from build123d import *

# Parameters (mm, degrees)
SKETCH1_W              = 215
SKETCH1_H              = 49
BOSS_EXTRUDE1_DEPTH    = 6
CUT_EXTRUDE1_REACH     = 141.058
SKETCH2_W              = 72
SKETCH2_H              = 6
SKETCH2_W_2            = 117
M8X1_25_TAPPED_HOLE1_D = 6.8
CUT_EXTRUDE2_REACH     = 141.058
SKETCH5_W              = 6
SKETCH5_H              = 20
SKETCH6_W              = 100
SKETCH6_H              = 6
BOSS_EXTRUDE2_DEPTH    = 6


with BuildPart() as part:
    # Sketch1 → Boss-Extrude1 (new body)
    with BuildSketch(Plane.XY):
        with Locations((-22.5, 24.5)):
            Rectangle(SKETCH1_W, SKETCH1_H)
    extrude(amount=BOSS_EXTRUDE1_DEPTH)

    # Sketch2 → Cut-Extrude1 (cut, up to next)
    with BuildSketch(Plane(origin=(0, 0, 0), x_dir=(-1, 0, 0), z_dir=(0, 0, -1)), mode=Mode.PRIVATE) as cut_extrude1_sk1:
        with Locations((-49, 46)):
            Rectangle(SKETCH2_W, SKETCH2_H)
    cut_extrude1_tool1 = extrude(cut_extrude1_sk1.sketch, amount=-CUT_EXTRUDE1_REACH, mode=Mode.PRIVATE) & part.part
    # Sketch2 → Cut-Extrude1 (cut, up to next)
    with BuildSketch(Plane(origin=(0, 0, 0), x_dir=(-1, 0, 0), z_dir=(0, 0, -1)), mode=Mode.PRIVATE) as cut_extrude1_sk2:
        with Locations((71.5, 46)):
            Rectangle(SKETCH2_W_2, SKETCH2_H)
    cut_extrude1_tool2 = extrude(cut_extrude1_sk2.sketch, amount=-CUT_EXTRUDE1_REACH, mode=Mode.PRIVATE) & part.part
    add(cut_extrude1_tool1.solids().sort_by_distance((49, 46, 0))[0], mode=Mode.SUBTRACT)
    add(cut_extrude1_tool2.solids().sort_by_distance((-71.5, 46, 0))[0], mode=Mode.SUBTRACT)

    # M8x1.25 Tapped Hole1 (through all)
    with Locations(Plane(origin=(0, 0, 0), x_dir=(-1, 0, 0), z_dir=(0, 0, -1))):
        with Locations((0, 39)):
            Hole(M8X1_25_TAPPED_HOLE1_D / 2)

    # Sketch5 → Cut-Extrude2 (cut, up to next)
    with BuildSketch(Plane(origin=(0, 0, 0), x_dir=(-1, 0, 0), z_dir=(0, 0, -1)), mode=Mode.PRIVATE) as cut_extrude2_sk1:
        with Locations((-82, 10)):
            Rectangle(SKETCH5_W, SKETCH5_H)
    cut_extrude2_tool1 = extrude(cut_extrude2_sk1.sketch, amount=-CUT_EXTRUDE2_REACH, mode=Mode.PRIVATE) & part.part
    # Sketch5 → Cut-Extrude2 (cut, up to next)
    with BuildSketch(Plane(origin=(0, 0, 0), x_dir=(-1, 0, 0), z_dir=(0, 0, -1)), mode=Mode.PRIVATE) as cut_extrude2_sk2:
        with Locations((127, 10)):
            Rectangle(SKETCH5_W, SKETCH5_H)
    cut_extrude2_tool2 = extrude(cut_extrude2_sk2.sketch, amount=-CUT_EXTRUDE2_REACH, mode=Mode.PRIVATE) & part.part
    add(cut_extrude2_tool1.solids().sort_by_distance((82, 10, 0))[0], mode=Mode.SUBTRACT)
    add(cut_extrude2_tool2.solids().sort_by_distance((-127, 10, 0))[0], mode=Mode.SUBTRACT)

    # Sketch6 → Boss-Extrude2 (add)
    with BuildSketch(Plane(origin=(0, 0, 0), x_dir=(-1, 0, 0), z_dir=(0, 0, -1))):
        with Locations((0, -3)):
            Rectangle(SKETCH6_W, SKETCH6_H)
    extrude(amount=-BOSS_EXTRUDE2_DEPTH)


solid = part.part
Design review of the part built by this model. Coordinates are the model's own, in mm. A direction names the side the tool comes from. Coordinates: 2 decimals unless noted, no trailing zeros. Loops run counter-clockwise (first coordinate to the right, second up) from the corner with the lowest first, then second, coordinate; pieces in that order, holes last. Notation, with made-up numbers: (-5, 50) -> (13, 50) arc R15 cw to (13, 75) -> close; hole circle Ø1 at (36.5, -39.75). An arc over 180 degrees is marked (long way). Use a Markdown table: item, result. Add a question column.
Item 1: We need section C-C, the plane z = 4.7. Write out the cut boundary in (x, y), and give its area (3 significant figures).
Item 2: We need section A-A, the plane y = 39. Write out the cut boundary in (x, z).
Item 3: Machinability: for faces 5 (the flat face through (-71, 43, 3)), 6 (the flat face through (64, 0, 3)), 7 (the flat face through (50, 43, 3)), 8 (the flat face through (-88, 0, 3)), which of the approach directions +Z, -Z, +X, -X, +Y, -Y give a long, thin tool a straight path to every point of the face, cutting with its end or side? Answer none if there is none.
Item 4: Clearance check with flat-ended pins moving along their axes: P1, Ø6, axis at x = 0, y = 39, coming from the +Z side; P2, Ø3, axis at x = -127.5, z = 2, coming from the -Y side; P3, Ø1, axis at y = 4.5, z = 1.5, coming from the +X side; P4, Ø1, axis at x = -84, z = 5, coming from the -Y side. State where each tip first meets the part, or that it passes through.
Item 5: We need section D-D, the plane x = -115.5. Write out the cut boundary in (y, z), and give its area (3 significant figures).
Item 6: Wall thickness on L1, parallel to Y at x = 0, z = 4.3; L2, parallel to Y at x = 37, z = 4.05; L3, parallel to X at y = 14, z = 4.5: over which ranges is each line inside the solid? List them lowest first. Write a range as from..to.
Item 7: We need section B-B, the plane x = 0. Write out the cut boundary in (y, z), and give its area (3 significant figures).
Item 8: The part is to be moulded in two halves that separate along X. For faces 1 (the flat face through (-50, -3, 3)), 2 (the flat face through (0, 49, 3)), 3 (the cylindrical face through (-0.44, 42.37, 3.04)), 4 (the flat face through (50, -3, 3)), say which applies: +X half, -X half, draft (parallel to the pull), parting line (faces both ways), or undercut.
Numbers:
| question | item | result |
|---|---|---|
| 1 | outline | (-130, 20) -> (-124, 20) -> (-124, 0) -> (-50, 0) -> (-50, -6) -> (50, -6) -> (50, 0) -> (79, 0) -> (79, 20) -> (85, 20) -> (85, 43) -> (13, 43) -> (13, 49) -> (-13, 49) -> (-13, 43) -> (-130, 43) -> close; hole circle Ø6.8 at (0, 39) |
| 1 | area | 9,720 mm^2 |
| 2 | outline | (-130, 0) -> (-3.4, 0) -> (-3.4, 6) -> (-130, 6) -> close; (3.4, 0) -> (85, 0) -> (85, 6) -> (3.4, 6) -> close |
| 3 | face 5 | +Z, -Z, -X, +Y |
| 3 | face 6 | +Z, -Z, +X, -Y |
| 3 | face 7 | +Z, -Z, +X, +Y |
| 3 | face 8 | +Z, -Z, -X, -Y |
| 4 | P1 | passes through |
| 4 | P2 | stops at y = 20 |
| 4 | P3 | stops at x = 79 |
| 4 | P4 | stops at y = 0 |
| 5 | outline | (0, 0) -> (43, 0) -> (43, 6) -> (0, 6) -> close |
| 5 | area | 258 mm^2 |
| 6 | L1 | y = -6..35.6, 42.4..49 |
| 6 | L2 | y = -6..43 |
| 6 | L3 | x = -124..79 |
| 7 | outline | (-6, 0) -> (35.6, 0) -> (35.6, 6) -> (-6, 6) -> close; (42.4, 0) -> (49, 0) -> (49, 6) -> (42.4, 6) -> close |
| 7 | area | 289 mm^2 |
| 8 | face 1 | -X half |
| 8 | face 2 | draft |
| 8 | face 3 | undercut |
| 8 | face 4 | +X half |
